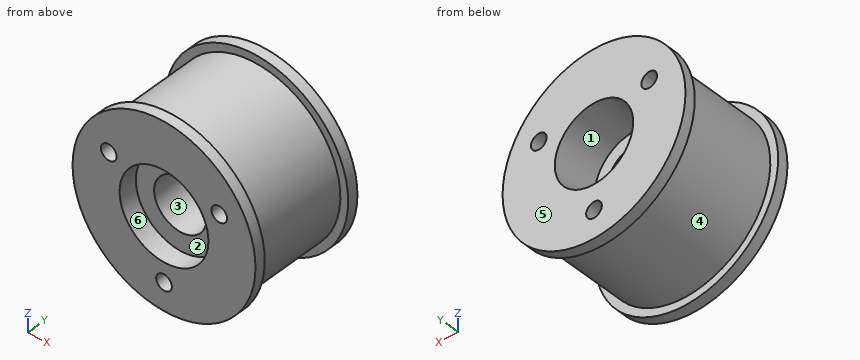
from build123d import *

# Parameters (mm, degrees)
SKETCH1_R                                           = 17.5
BOSS_EXTRUDE1_DEPTH                                 = 22
CBORE_FOR_M8_HEX_SOCKET_HEAD_CAP_SCREW1_D           = 10
CBORE_FOR_M8_HEX_SOCKET_HEAD_CAP_SCREW1_CBORE_D     = 15
CBORE_FOR_M8_HEX_SOCKET_HEAD_CAP_SCREW1_CBORE_DEPTH = 8.6
F_3_0MM_DOWEL_HOLE1_D                               = 3
SKETCH6_R                                           = 8.5
CUT_EXTRUDE1_DEPTH                                  = 3.5
CUT_EXTRUDE2_START                                  = -2
SKETCH7_R                                           = 17.5
SKETCH7_R_2                                         = 16
CUT_EXTRUDE2_DEPTH                                  = 18


with BuildPart() as part:
    # Sketch1 → Boss-Extrude1 (new body)
    with BuildSketch(Plane(origin=(0, 0, 0), x_dir=(1, 0, 0), z_dir=(0, 1, 0))):
        with Locations(Location((0, 0, 0), (0, 0, 270))):
            Circle(SKETCH1_R)
    extrude(amount=BOSS_EXTRUDE1_DEPTH)

    # CBORE for M8 Hex Socket Head Cap Screw1 (through all)
    with Locations(Plane(origin=(0, 22, 0), x_dir=(1, 0, 0), z_dir=(0, 1, 0))):
        with Locations((0, 0)):
            CounterBoreHole(CBORE_FOR_M8_HEX_SOCKET_HEAD_CAP_SCREW1_D / 2, CBORE_FOR_M8_HEX_SOCKET_HEAD_CAP_SCREW1_CBORE_D / 2, CBORE_FOR_M8_HEX_SOCKET_HEAD_CAP_SCREW1_CBORE_DEPTH)

    # Ø3.0mm Dowel Hole1 (through all)
    with Locations(Plane(origin=(0, 22, 0), x_dir=(1, 0, 0), z_dir=(0, 1, 0))):
        with Locations((-10.565509926, -6.1), (0, 12.2), (10.565509926, -6.1)):
            Hole(F_3_0MM_DOWEL_HOLE1_D / 2)

    # Sketch6 → Cut-Extrude1 (cut)
    with BuildSketch(Plane.XZ):
        with Locations(Location((0, 0, 0), (0, 0, 270))):
            Circle(SKETCH6_R)
    extrude(amount=-CUT_EXTRUDE1_DEPTH, mode=Mode.SUBTRACT)

    # Sketch7 → Cut-Extrude2 (cut)
    with BuildSketch(Plane.XZ.offset(CUT_EXTRUDE2_START)):
        with Locations(Location((0, 0, 0), (0, 0, 270))):
            Circle(SKETCH7_R)
        with Locations(Location((0, 0, 0), (0, 0, 270))):
            Circle(SKETCH7_R_2, mode=Mode.SUBTRACT)
    extrude(amount=-CUT_EXTRUDE2_DEPTH, mode=Mode.SUBTRACT)


solid = part.part
Input: part model. Units: mm. Frame: model coordinates. Face numbers are marked on the shaded views. A direction names the side the tool comes from. Round coordinates to 2 decimals unless told otherwise and drop trailing zeros. Loops run counter-clockwise (first coordinate to the right, second up) from the corner with the lowest first, then second, coordinate; pieces in that order, holes last. Notation, with made-up numbers: M 39.25,43 L 50.25,43 A28 ccw 50.25,76 Z; hole C 59,-15.5 d3. An arc over 180 degrees is marked long. Answer as CSV lines item,"result". Start each with the question number.
(1) Section D-D, the plane z = 7. Output: boundary loops of the cut face in (x, y).
(2) Section A-A, the plane z = 0. Output: boundary loops of the cut face in (x, y).
(3) First-contact query: pin 1 (11.5 mm diameter, centred on x = 0, z = 0, fed in from +Y); pin 2 (6 mm diameter, centred on x = -9.5, y = 6.5, fed in from +Z); pin 3 (8 mm diameter, centred on x = -13, y = 13, fed in from -Z). Flat tips, straight axial feed; report the tip coordinate or a pass-through.
(4) Section B-B, the plane y = 4.5. Output: boundary loops of the cut face in (x, z), plus the area to 3 significant figures.
(5) Reachability of the marked faces 1, 2 and 3 from +Z, -Z, +X, -X, +Y, -Y: full face, straight path, thin tool, end or side. Return the list, or none.
(6) Draft query along Y for the marked faces 4, 5 and 6. Return one class per face: released by +Y, released by -Y, zero draft, split by the parting line, or undercut.
(7) Section C-C, the plane x = 4. Output: boundary loops of the cut face in (y, z), plus the area to 3 significant figures.
(8) Line query: line 1 (Y direction, x = -9, z = 14); line 2 (X direction, y = 2.35, z = 0); line 3 (X direction, y = 14.5, z = 6.1). Output: solid intervals per line, ascending. Write a range as [from, to].
Values found:
1,outline,"M -16.04,0 L -11.77,0 L -11.77,22 L -16.04,22 L -16.04,20 L -14.39,20 L -14.39,2 L -16.04,2 Z; M -9.37,0 L -4.82,0 L -4.82,3.5 L 4.82,3.5 L 4.82,0 L 9.37,0 L 9.37,22 L 2.69,22 L 2.69,13.4 L -2.69,13.4 L -2.69,22 L -9.37,22 Z; M 11.77,0 L 16.04,0 L 16.04,2 L 14.39,2 L 14.39,20 L 16.04,20 L 16.04,22 L 11.77,22 Z"
2,outline,"M -17.5,0 L -8.5,0 L -8.5,3.5 L -5,3.5 L -5,13.4 L -7.5,13.4 L -7.5,22 L -17.5,22 L -17.5,20 L -16,20 L -16,2 L -17.5,2 Z; M 5,3.5 L 8.5,3.5 L 8.5,0 L 17.5,0 L 17.5,2 L 16,2 L 16,20 L 17.5,20 L 17.5,22 L 7.5,22 L 7.5,13.4 L 5,13.4 Z"
3,pin 1,"stops at y = 13.4"
3,pin 2,"stops at z = 14.62"
3,pin 3,"stops at z = -13.23"
4,outline,"C 0,0 d32; hole C -10.57,6.1 d3; hole C 0,0 d10; hole C 0,-12.2 d3; hole C 10.57,6.1 d3"
4,area,"705 mm²"
5,face 1,"+Y"
5,face 2,"-Y"
5,face 3,"+Y, -Y"
6,face 4,"undercut"
6,face 5,"released by +Y"
6,face 6,"zero draft"
7,outline,"M 0,-17.04 L 2,-17.04 L 2,-15.49 L 20,-15.49 L 20,-17.04 L 22,-17.04 L 22,-6.34 L 13.4,-6.34 L 13.4,-3 L 3.5,-3 L 3.5,-7.5 L 0,-7.5 Z; M 0,7.5 L 3.5,7.5 L 3.5,3 L 13.4,3 L 13.4,6.34 L 22,6.34 L 22,17.04 L 20,17.04 L 20,15.49 L 2,15.49 L 2,17.04 L 0,17.04 Z"
7,area,"473 mm²"
8,line 1,"y = [0, 2], [20, 22]"
8,line 2,"x = [-16, -8.5], [8.5, 16]"
8,line 3,"x = [-14.79, -12.07], [-9.07, -4.36], [4.36, 9.07], [12.07, 14.79]"
